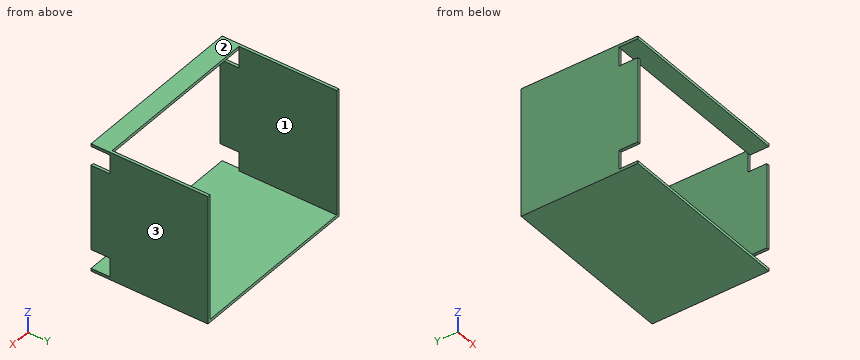
from build123d import *

# Parameters (mm, degrees)
SKETCH2_W               = 186
SKETCH2_H               = 136
BOSS_EXTRUDE1_DEPTH     = 20
BOSS_EXTRUDE2_DEPTH     = 103
CUT_EXTRUDE1_DEPTH      = 224.224102641
CUT_EXTRUDE1_DEPTH_BACK = 224.224102641
SKETCH4_W               = 20
SKETCH4_H               = 20


with BuildPart() as part:
    # Sketch2 → Boss-Extrude1 (new body)
    with BuildSketch(Plane(origin=(0, 0, 0), x_dir=(1, 0, 0), z_dir=(0, 1, 0))):
        Rectangle(SKETCH2_W, SKETCH2_H)
        Polygon((-90, -65), (-90, -60), (-90, 60), (-90, 65), (90, 65), (90, 60), (90, -60), (90, -65), align=None, mode=Mode.SUBTRACT)
    extrude(amount=-BOSS_EXTRUDE1_DEPTH)

    # Sketch3 → Boss-Extrude2 (add)
    with BuildSketch(Plane(origin=(0, 0, 0), x_dir=(1, 0, 0), z_dir=(0, 1, 0))):
        Polygon((-93, 65), (-93, -68), (-90, -68), (-90, -65), (-90, 65), align=None)
        Polygon((-93, 68), (-93, 65), (-90, 65), (90, 65), (93, 65), (93, 68), align=None)
        Polygon((90, -65), (90, -68), (93, -68), (93, 65), (90, 65), align=None)
    extrude(amount=BOSS_EXTRUDE2_DEPTH)

    # Sketch4 → Cut-Extrude1 (cut, two sides: drawn at the far end of the back side and taken through both)
    with BuildSketch(Plane(origin=(93, 0, 0), x_dir=(0, 0, -1), z_dir=(1, 0, 0)).offset(-CUT_EXTRUDE1_DEPTH_BACK)):
        with Locations((-55, -10)):
            Rectangle(SKETCH4_W, SKETCH4_H)
        with Locations((55, -10)):
            Rectangle(SKETCH4_W, SKETCH4_H)
    extrude(amount=CUT_EXTRUDE1_DEPTH + CUT_EXTRUDE1_DEPTH_BACK, mode=Mode.SUBTRACT)


solid = part.part
Check sheet for the modelled part. Datum: model origin and axes. Units: mm. Face numbers are marked on the shaded views. Give positions to 0.01 mm unless a question says otherwise; leave off trailing zeros. Loops run counter-clockwise (first coordinate to the right, second up) from the corner with the lowest first, then second, coordinate; pieces in that order, holes last. Notation, with made-up numbers: M 46.25,66 L 66.25,66 A23 ccw 66.25,75 Z; hole C 88,29.25 d9. An arc over 180 degrees is marked long. Answer as a JSON object with one key per item and string values. Group by question number.
Q1. Go/stop test with flat-tipped pins: P1, Ø0.9, axis at x = -91.5, z = 58, coming from the -Y side; P2, Ø2.5, axis at x = -1, z = 66, coming from the +Y side. Record where each tip stops, or that it passes through.
Q2. Cross-section at C-C on y = 22. Record the cut outline in (x, z).
Q3. Material ranges on line 1 along X through (y, z) = (31.5, -53.5); line 2 along Z through (x, y) = (49, -3); line 3 along Z through (x, y) = (-37.5, 9), recorded low to high. Write a range as [from, to].
Q4. Release check for a two-part mould opening along X. For the marked faces 1, 2 and 3 record: released by +X, released by -X, zero draft, split by the parting line, or undercut.
Q5. Cross-section at A-A on x = 76. Record the cut outline in (y, z), then the cut area to 3 significant figures.
Q6. Cross-section at B-B on z = 12. Record the cut outline in (x, y).
Evaluation:
{
 "1": {"P1": "stops at y = 0", "P2": "stops at y = 0"},
 "2": {"outline": "M -93,-68 L 93,-68 L 93,68 L 90,68 L 90,-65 L -90,-65 L -90,68 L -93,68 Z"},
 "3": {"line 1": "x = [-93, -90], [90, 93]", "line 2": "z = [-68, -65], [65, 68]", "line 3": "z = [-68, -65]"},
 "4": {"face 1": "undercut", "face 2": "zero draft", "face 3": "released by +X"},
 "5": {"outline": "M -20,-68 L 103,-68 L 103,-65 L -20,-65 Z; M -20,65 L 0,65 L 0,68 L -20,68 Z", "area": "429 mm2"},
 "6": {"outline": "M -93,-20 L -90,-20 L -90,103 L -93,103 Z; M 90,-20 L 93,-20 L 93,103 L 90,103 Z"}
}
